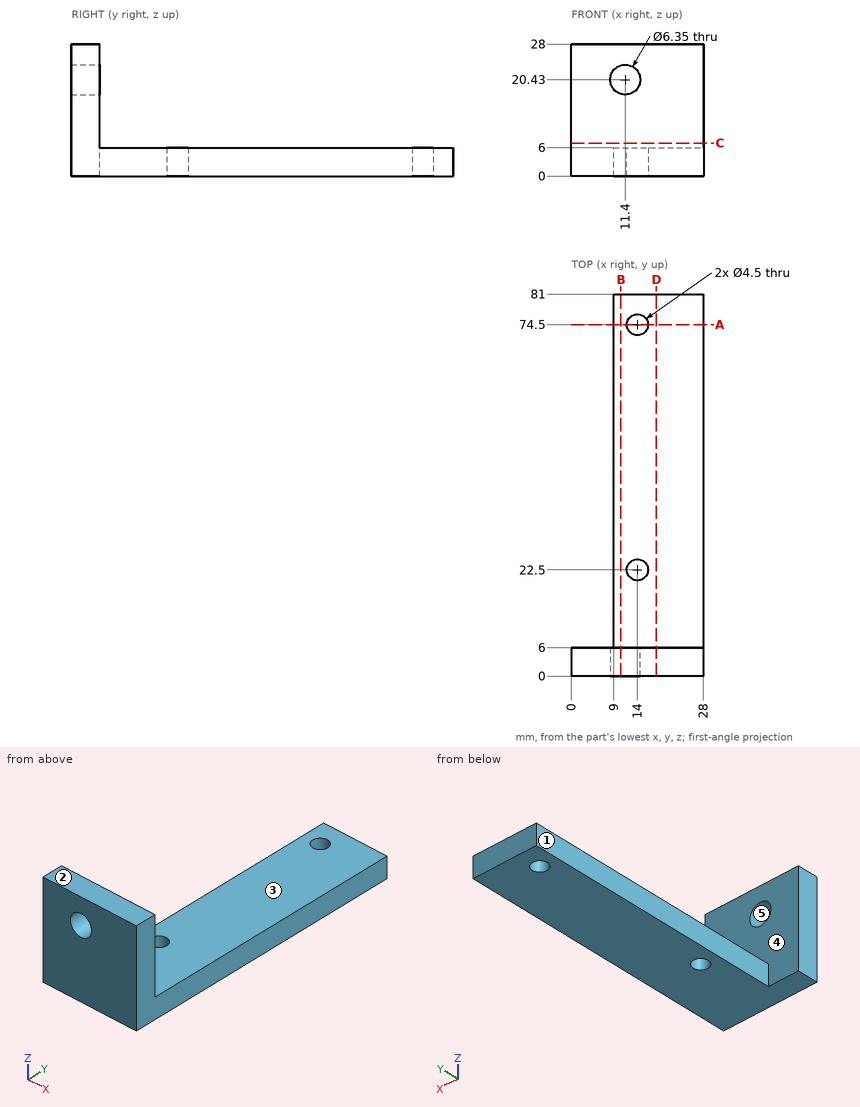
Verification items for this drawing (mm, ordinates from the low corner). A direction names the side the tool comes from. Coordinates: 2 decimals unless noted, no trailing zeros. Write each loop counter-clockwise with the first axis right and the second up, starting at its lowest first coordinate (ties: lowest second). Pieces come first, ordered by that corner, then holes. Notation, with made-up numbers: M 50,-39 L 58,-39 A23 cw 58,-8 Z; hole C 53.5,-37 d6. An arc over 180 degrees is marked long. Use one line per item in the form item = value. Start each with the question number.
1) Go/stop test with flat-tipped pins: pin 1 Ø1.8 at (y, z) = (36, 3) entering from -X; pin 2 Ø5.5 at (x, y) = (19, 40.5) entering from +Z; pin 3 Ø8 at (x, y) = (24, 38) entering from -Z. Record where each tip stops, or that it passes through.
2) Release check for a two-part mould opening along Z. For the marked faces 3, 4 and 5 record: pulls with the +Z half, pulls with the -Z half, needs draft (parallel to the pull), parting line crosses it, or undercut.
3) Section check A-A on y = 74.5. Enter the section's corners in (x, z), and give its area (3 significant figures).
4) Thickness scan on probe 1 along Y at (x, z) = (14, 3); probe 2 along Z at (x, y) = (11.4, 1.9) (3 decimals); probe 3 along X at (y, z) = (74.5, 3). Record the ranges inside material, lowest first. Write a range as from..to.
5) Section check D-D on x = 18. Enter the section's corners in (y, z).
6) Section check C-C on z = 7. Enter the section's corners in (x, y).
7) Set-up check for the marked faces 1 and 2: record each of +Z, -Z, +X, -X, +Y, -Y from which the full face is reachable in a straight line by a thin tool's end or side.
8) Section check B-B on x = 10.5. Enter the section's corners in (y, z), and give its area (3 significant figures).
Responses:
q1.pin_1 = 9
q1.pin_2 = 6
q1.pin_3 = 0
q2.face_3 = pulls with the +Z half
q2.face_4 = needs draft
q2.face_5 = undercut
q3.outline = M 9,0 L 11.75,0 L 11.75,6 L 9,6 Z; M 16.25,0 L 28,0 L 28,6 L 16.25,6 Z
q3.area = 87.0 mm2
q4.probe_1 = 0..20.25, 24.75..72.25, 76.75..81
q4.probe_2 = 0..17.255, 23.605..28
q4.probe_3 = 9..11.75, 16.25..28
q5.outline = M 0,0 L 81,0 L 81,6 L 6,6 L 6,28 L 0,28 Z
q6.outline = M 0,0 L 28,0 L 28,6 L 0,6 Z
q7.face_1 = +Z, -Z, -X, +Y
q7.face_2 = +Z, +X, -X, +Y, -Y
q8.outline = M 0,0 L 81,0 L 81,6 L 6,6 L 6,17.39 L 0,17.39 Z; M 0,23.47 L 6,23.47 L 6,28 L 0,28 Z
q8.area = 581 mm2
